Autodesk Inventor part; units mm, degrees
ref_plane "YZ Plane" through (0, 0, 0) normal (1, 0, 0) x (0, 1, 0)
ref_plane "XZ Plane" through (0, 0, 0) normal (0, 1, 0) x (-1, 0, 0)
ref_plane "XY Plane" through (0, 0, 0) normal (0, 0, 1) x (1, 0, 0)
sketch "Sketch1" plane through (0, 0, 0) normal (0, 0, 1) x (1, 0, 0)
  line L0 (-25.4, -88.9) -> (25.4, -88.9)
  line L1 (25.4, -88.9) -> (25.4, 88.9)
  line L2 (25.4, 88.9) -> (-25.4, 88.9)
  line L3 (-25.4, 88.9) -> (-25.4, -88.9)
  line L4 (-25.4, -88.9) -> (25.4, 88.9) construction
  line L5 (25.4, -88.9) -> (-25.4, 88.9) construction
  point P0 (0, 0)
  dimension "width" = 50.8
  dimension "length" = 177.8
extrude "Extrusion1" add sketch "Sketch1" along normal mid plane 6.35
sketch "Sketch2" plane through (0, 0, 3.175) normal (0, 0, 1) x (1, 0, 0)
  line L0 (-25.4, -88.9) -> (-25.4, 88.9) construction
  line L1 (-25.4, 88.9) -> (25.4, 88.9) construction
  line L2 (25.4, 88.9) -> (25.4, -88.9) construction
  line L3 (25.4, -88.9) -> (-25.4, -88.9) construction
  point P0 (0, 0)
  point P1 (0, -63.5)
  point P2 (0, -88.9)
  dimension "d4" = 25.4
hole "Hole1" at (0, -63.5, 3.175) direction (0, 0, -1) diameter 28.575 end through all
properties part number "CL6-003" material "Aluminum 6061"
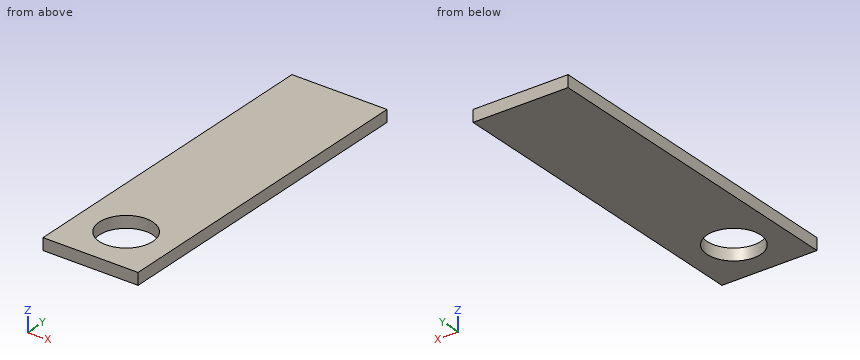
The model under review builds one solid part; all positions refer to its coordinate system, in mm. Round coordinates to 2 decimals unless told otherwise and drop trailing zeros. Write each loop counter-clockwise with the first axis right and the second up, starting at its lowest first coordinate (ties: lowest second). Pieces come first, ordered by that corner, then holes.
(1) We need section A-A on x = 0. Give the boundary of the cut face in (y, z) (1 decimal).
(2) We need section C-C on z = 1. Give the boundary of the cut face in (x, y) (1 decimal).
(3) Wall thickness on L1, parallel to X at y = -63.5, z = -1.5; L2, parallel to Y at x = 0, z = -1.5; L3, parallel to Y at x = -6, z = 0.5: over which ranges is each line inside the solid? List them lowest first.
(4) We need section B-B on y = -63.5. Give the boundary of the cut face in (x, z) (1 decimal), and give its area (3 significant figures).
Findings below:
1. outline: (-88.9, -3.2) - (-77.8, -3.2) - (-77.8, 3.2) - (-88.9, 3.2) - close; (-49.2, -3.2) - (88.9, -3.2) - (88.9, 3.2) - (-49.2, 3.2) - close
2. outline: (-25.4, -88.9) - (25.4, -88.9) - (25.4, 88.9) - (-25.4, 88.9) - close; hole circle Ø28.6 at (0, -63.5)
3. L1: x = -25.4 to -14.29, 14.29 to 25.4
3. L2: y = -88.9 to -77.79, -49.21 to 88.9
3. L3: y = -88.9 to -76.47, -50.53 to 88.9
4. outline: (-25.4, -3.2) - (-14.3, -3.2) - (-14.3, 3.2) - (-25.4, 3.2) - close; (14.3, -3.2) - (25.4, -3.2) - (25.4, 3.2) - (14.3, 3.2) - close
4. area: 141 mm2
